Geometry: final body of the model. Coordinates: model frame, mm. Face numbers are marked on the shaded views. Coordinates: 2 decimals unless noted, no trailing zeros. Write each loop counter-clockwise with the first axis right and the second up, starting at its lowest first coordinate (ties: lowest second). Pieces come first, ordered by that corner, then holes.
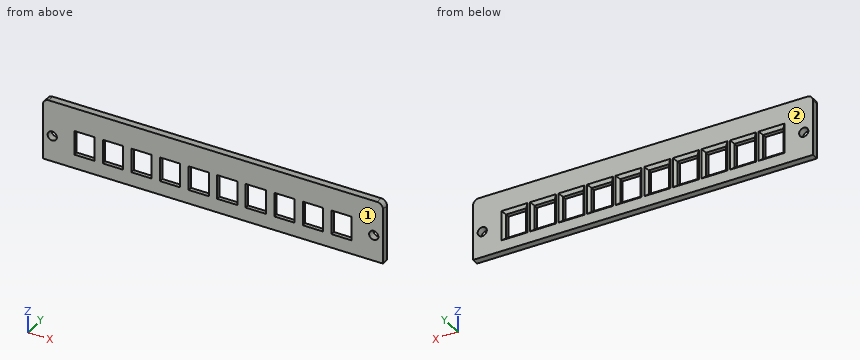
Autodesk Inventor part; units mm, degrees
ref_plane "YZ Plane" through (0, 0, 0) normal (1, 0, 0) x (0, 1, 0)
ref_plane "XZ Plane" through (0, 0, 0) normal (0, 1, 0) x (-1, 0, 0)
ref_plane "XY Plane" through (0, 0, 0) normal (0, 0, 1) x (1, 0, 0)
sketch "Sketch1" plane through (0, 0, 0) normal (0, 1, 0) x (-1, 0, 0)
  line L0 (0, 0) -> (-9.9, 0)
  line L1 (0, 0) -> (0, -10.3)
  line L2 (0, -10.3) -> (-9.9, -10.3)
  line L3 (-9.9, -10.3) -> (-9.9, 0)
  line L4 (-9.9, -10.3) -> (-9.4, -10.3)
  line L5 (-9.4, -10.3) -> (-9.4, 0)
  line L6 (0, -10.3) -> (-0.5, -10.3)
  line L7 (-0.5, -10.3) -> (-0.5, 0)
  line L8 (-0.5, 0.85) -> (-9.9, 0.85)
  line L9 (-9.9, 0.85) -> (-9.9, 0)
  line L10 (0, 0) -> (0, 0.85)
  line L11 (0, 0.85) -> (-0.5, 0.85)
  line L12 (0, -10.3) -> (0, -11.15)
  line L13 (0, -11.15) -> (-9.9, -11.15)
  line L14 (-9.9, -11.15) -> (-9.9, -10.3)
  line L15 (-9.9, -11.15) -> (-19.8, -11.15)
  line L16 (-19.8, -11.15) -> (-19.8, -10.3)
  line L17 (-19.8, -10.3) -> (-19.8, 0)
  line L18 (-19.3, -10.3) -> (-19.3, 0)
  line L19 (-9.9, -10.3) -> (-19.8, -10.3)
  line L20 (-10.4, -10.3) -> (-10.4, 0)
  line L21 (-9.9, 0) -> (-9.9, -10.3)
  line L22 (-9.9, 0) -> (-9.9, 0.85)
  line L23 (-9.9, 0.85) -> (-10.4, 0.85)
  line L24 (-10.4, 0.85) -> (-19.8, 0.85)
  line L25 (-9.9, 0) -> (-19.8, 0)
  line L26 (-19.8, 0.85) -> (-19.8, 0)
  line L27 (-19.8, -11.15) -> (-29.7, -11.15)
  line L28 (-29.7, -11.15) -> (-29.7, -10.3)
  line L29 (-29.7, -10.3) -> (-29.7, 0)
  line L30 (-29.2, -10.3) -> (-29.2, 0)
  line L31 (-19.8, -10.3) -> (-29.7, -10.3)
  line L32 (-20.3, -10.3) -> (-20.3, 0)
  line L33 (-19.8, 0) -> (-19.8, -10.3)
  line L34 (-19.8, 0) -> (-19.8, 0.85)
  line L35 (-19.8, 0.85) -> (-20.3, 0.85)
  line L36 (-20.3, 0.85) -> (-29.7, 0.85)
  line L37 (-19.8, 0) -> (-29.7, 0)
  line L38 (-29.7, 0.85) -> (-29.7, 0)
  line L39 (-29.7, -11.15) -> (-39.6, -11.15)
  line L40 (-39.6, -11.15) -> (-39.6, -10.3)
  line L41 (-39.6, -10.3) -> (-39.6, 0)
  line L42 (-39.1, -10.3) -> (-39.1, 0)
  line L43 (-29.7, -10.3) -> (-39.6, -10.3)
  line L44 (-30.2, -10.3) -> (-30.2, 0)
  line L45 (-29.7, 0) -> (-29.7, -10.3)
  line L46 (-29.7, 0) -> (-29.7, 0.85)
  line L47 (-29.7, 0.85) -> (-30.2, 0.85)
  line L48 (-30.2, 0.85) -> (-39.6, 0.85)
  line L49 (-29.7, 0) -> (-39.6, 0)
  line L50 (-39.6, 0.85) -> (-39.6, 0)
  line L51 (-39.6, -11.15) -> (-49.5, -11.15)
  line L52 (-49.5, -11.15) -> (-49.5, -10.3)
  line L53 (-49.5, -10.3) -> (-49.5, 0)
  line L54 (-49, -10.3) -> (-49, 0)
  line L55 (-39.6, -10.3) -> (-49.5, -10.3)
  line L56 (-40.1, -10.3) -> (-40.1, 0)
  line L57 (-39.6, 0) -> (-39.6, -10.3)
  line L58 (-39.6, 0) -> (-39.6, 0.85)
  line L59 (-39.6, 0.85) -> (-40.1, 0.85)
  line L60 (-40.1, 0.85) -> (-49.5, 0.85)
  line L61 (-39.6, 0) -> (-49.5, 0)
  line L62 (-49.5, 0.85) -> (-49.5, 0)
  line L63 (-49.5, -11.15) -> (-59.4, -11.15)
  line L64 (-59.4, -11.15) -> (-59.4, -10.3)
  line L65 (-59.4, -10.3) -> (-59.4, 0)
  line L66 (-58.9, -10.3) -> (-58.9, 0)
  line L67 (-49.5, -10.3) -> (-59.4, -10.3)
  line L68 (-50, -10.3) -> (-50, 0)
  line L69 (-49.5, 0) -> (-49.5, -10.3)
  line L70 (-49.5, 0) -> (-49.5, 0.85)
  line L71 (-49.5, 0.85) -> (-50, 0.85)
  line L72 (-50, 0.85) -> (-59.4, 0.85)
  line L73 (-49.5, 0) -> (-59.4, 0)
  line L74 (-59.4, 0.85) -> (-59.4, 0)
  line L75 (-59.4, -11.15) -> (-69.3, -11.15)
  line L76 (-69.3, -11.15) -> (-69.3, -10.3)
  line L77 (-69.3, -10.3) -> (-69.3, 0)
  line L78 (-68.8, -10.3) -> (-68.8, 0)
  line L79 (-59.4, -10.3) -> (-69.3, -10.3)
  line L80 (-59.9, -10.3) -> (-59.9, 0)
  line L81 (-59.4, 0) -> (-59.4, -10.3)
  line L82 (-59.4, 0) -> (-59.4, 0.85)
  line L83 (-59.4, 0.85) -> (-59.9, 0.85)
  line L84 (-59.9, 0.85) -> (-69.3, 0.85)
  line L85 (-59.4, 0) -> (-69.3, 0)
  line L86 (-69.3, 0.85) -> (-69.3, 0)
  line L87 (-69.3, -11.15) -> (-79.2, -11.15)
  line L88 (-79.2, -11.15) -> (-79.2, -10.3)
  line L89 (-79.2, -10.3) -> (-79.2, 0)
  line L90 (-78.7, -10.3) -> (-78.7, 0)
  line L91 (-69.3, -10.3) -> (-79.2, -10.3)
  line L92 (-69.8, -10.3) -> (-69.8, 0)
  line L93 (-69.3, 0) -> (-69.3, -10.3)
  line L94 (-69.3, 0) -> (-69.3, 0.85)
  line L95 (-69.3, 0.85) -> (-69.8, 0.85)
  line L96 (-69.8, 0.85) -> (-79.2, 0.85)
  line L97 (-69.3, 0) -> (-79.2, 0)
  line L98 (-79.2, 0.85) -> (-79.2, 0)
  line L99 (-79.2, -11.15) -> (-89.1, -11.15)
  line L100 (-89.1, -11.15) -> (-89.1, -10.3)
  line L101 (-89.1, -10.3) -> (-89.1, 0)
  line L102 (-88.6, -10.3) -> (-88.6, 0)
  line L103 (-79.2, -10.3) -> (-89.1, -10.3)
  line L104 (-79.7, -10.3) -> (-79.7, 0)
  line L105 (-79.2, 0) -> (-79.2, -10.3)
  line L106 (-79.2, 0) -> (-79.2, 0.85)
  line L107 (-79.2, 0.85) -> (-79.7, 0.85)
  line L108 (-79.7, 0.85) -> (-89.1, 0.85)
  line L109 (-79.2, 0) -> (-89.1, 0)
  line L110 (-89.1, 0.85) -> (-89.1, 0)
  line L111 (-89.1, -11.15) -> (-99, -11.15)
  line L112 (-99, -11.15) -> (-99, -10.3)
  line L113 (-99, -10.3) -> (-99, 0)
  line L114 (-98.5, -10.3) -> (-98.5, 0)
  line L115 (-89.1, -10.3) -> (-99, -10.3)
  line L116 (-89.6, -10.3) -> (-89.6, 0)
  line L117 (-89.1, 0) -> (-89.1, -10.3)
  line L118 (-89.1, 0) -> (-89.1, 0.85)
  line L119 (-89.1, 0.85) -> (-89.6, 0.85)
  line L120 (-89.6, 0.85) -> (-99, 0.85)
  line L121 (-89.1, 0) -> (-99, 0)
  line L122 (-99, 0.85) -> (-99, 0)
  line L123 (0, -11.15) -> (0, 0.85)
  line L124 (0, -11.15) -> (0, -14.15)
  line L125 (0, -14.15) -> (0, -14.15)
  line L126 (-99, 0.85) -> (-102, 0.85)
  line L127 (-102, 0.85) -> (-102, 3.85)
  line L128 (0, -14.15) -> (-102, -14.15)
  line L129 (-102, -14.15) -> (-102, 3.85)
  line L130 (0, 3.89) -> (0, -14.15)
  line L131 (0, -11.15) -> (0, -11.15)
  line L132 (0, 0.85) -> (0, 0.85)
  line L133 (0, -11.15) -> (-2, -11.15)
  line L134 (-2, -11.15) -> (-2, 0.85)
  line L135 (0, -14.15) -> (3.2, -14.15)
  line L136 (3.2, -14.15) -> (3.2, 3.89)
  line L137 (3.2, 3.89) -> (0, 3.89)
  line L138 (0, -11.15) -> (3.2, -11.15)
  line L139 (0, 0.85) -> (3.2, 0.85)
  line L140 (3.2, -14.15) -> (6.2, -14.15)
  line L141 (6.2, 3.89) -> (3.2, 3.89)
  line L142 (0, -14.15) -> (6.2, -14.15)
  line L143 (-49.5, 3.85) -> (-49.5, 0.85)
  line L144 (6.2, 3.89) -> (6.2, 7.09)
  line L145 (6.2, 7.09) -> (6.2, 13.49)
  line L146 (3.2, 3.89) -> (3.2, 13.45)
  line L147 (-102, 3.85) -> (-102, 13.45)
  line L148 (0, 3.89) -> (0, 13.49)
  line L149 (-49.5, 3.85) -> (-87.8335, 3.85)
  line L150 (-49.5, 3.85) -> (-11.1665, 3.89)
  line L151 (-11.1665, 3.89) -> (0, 3.89)
  line L152 (-87.8335, 3.85) -> (-102, 3.85)
  line L153 (-102, -14.15) -> (-105, -14.15)
  line L154 (-105, 13.49) -> (6.2, 13.49)
  line L155 (6.2, 7.09) -> (-105, 7.09)
  line L156 (-49.5, 3.85) -> (-49.5, 7.09)
  line L157 (-49.5, 7.09) -> (-49.5, 10.29)
  line L158 (-49.5, 10.29) -> (-11.1665, 10.29)
  line L159 (-49.5, 10.29) -> (-87.8335, 10.29)
  line L160 (-91.0335, 13.49) -> (-84.6335, 13.49)
  line L161 (-84.6335, 13.49) -> (-84.6335, 7.09)
  line L162 (-84.6335, 7.09) -> (-91.0335, 7.09)
  line L163 (-91.0335, 7.09) -> (-91.0335, 13.49)
  line L164 (-91.0335, 13.49) -> (-84.6335, 7.09) construction
  line L165 (-84.6335, 13.49) -> (-91.0335, 7.09) construction
  line L166 (-14.3665, 13.49) -> (-7.9665, 13.49)
  line L167 (-7.9665, 13.49) -> (-7.9665, 7.09)
  line L168 (-7.9665, 7.09) -> (-14.3665, 7.09)
  line L169 (-14.3665, 7.09) -> (-14.3665, 13.49)
  line L170 (-14.3665, 13.49) -> (-7.9665, 7.09) construction
  line L171 (-7.9665, 13.49) -> (-14.3665, 7.09) construction
  circle A0 centre (-11.1665, 10.29) radius 1.6
  circle A1 centre (-87.8335, 10.29) radius 1.6
  line L172 (6.2, -14.15) -> (9.4, -14.15)
  line L173 (9.4, -14.15) -> (9.4, 3.89)
  line L174 (9.4, 3.89) -> (6.2, 3.89)
  line L175 (9.4, 3.89) -> (9.4, 7.09)
  line L176 (9.4, 7.09) -> (6.2, 7.09)
  line L177 (-105, 7.09) -> (-108.2, 7.09)
  line L178 (-108.2, -14.15) -> (-105, -14.15)
  line L179 (-105, 13.49) -> (-105, 7.09)
  line L180 (-102, -14.15) -> (-108.4, -14.15)
  line L181 (-108.4, -14.15) -> (-108.4, 7.09)
  line L182 (-108.4, 7.09) -> (-108.2, 7.09)
  line L183 (-108.4, -5.13) -> (-105.2, -5.13)
  line L184 (3.2, -11.15) -> (3.2, 0.85)
  line L185 (3.2, -5.15) -> (9.4, -5.15)
  line L186 (3.2, -5.15) -> (9.4, -5.15) construction
  line L187 (9.4, -5.15) -> (6.2, -5.15)
  circle A2 centre (6.2, -5.15) radius 1.6
  circle A3 centre (-105.2, -5.15) radius 1.6
  line L188 (0, 0) -> (-9.9, 0)
  line L189 (-4.95, 0) -> (-4.95, -10.3)
  line L190 (-8.45, -0.95) -> (-1.45, -0.95)
  line L191 (-1.45, -0.95) -> (-1.45, -9.35)
  line L192 (-1.45, -9.35) -> (-8.45, -9.35)
  line L193 (-8.45, -9.35) -> (-8.45, -0.95)
  line L194 (-8.45, -0.95) -> (-1.45, -9.35) construction
  line L195 (-1.45, -0.95) -> (-8.45, -9.35) construction
  line L196 (-9.4, 0) -> (-0.5, 0)
  point P0 (-2, 0)
  point P1 (-2, -10.3)
  point P2 (0, 0.85)
  point P3 (0, 7.09)
  point P4 (3.2, 7.09)
  point P5 (-4.95, -5.15)
  dimension "d0" = 9.9
  dimension "d1" = 10.3
  dimension "d2" = 0.5
  dimension "d3" = 0.5
  dimension "d6" = 0.85
  dimension "d7" = 0.85
  dimension "d10" = 9.9
  dimension "d15" = 3
  dimension "d16" = 0
  dimension "d19" = 3
  dimension "d20" = 2
  dimension "d30" = 3.2
  dimension "d31" = 3
  dimension "d32" = 3
  dimension "d35" = 3.2
  dimension "d36" = 6.4
  dimension "d38" = 38.3335
  dimension "d45" = 3.2
  dimension "d47" = 38.3335
  dimension "d48" = 6.4
  dimension "d49" = 6.4
  dimension "d50" = 3.2
  dimension "d51" = 3.2
  dimension "d53" = 6.4
  dimension "d58" = 3.2
  dimension "d59" = 3.2
  dimension "d60" = 3.2
  dimension "d63" = 7
  dimension "d64" = 8.4
  dimension "d72" = 8.9
extrude "Extrusion6" add sketch "Sketch1" along normal blind 2.4 contours L1 L2 L7 L0 | L10 L139 L136 L138 L12 L1 | L0 L134 L8 L11 L10 | L7 L2 L134 L192 L191 L190 L0 | L12 L13 L134 L2 | L11 L8 L23 L24 L35 L36 L47 L48 L59 L60 L143 L150 L151 L130 | L130 L137 L136 L139 | L134 L190 L189 L0 | L0 L9 L8 L134 | L124 L128 L129 L126 L122 L113 L112 L111 L99 L87 L75 L63 L51 L39 L27 L15 L13 | L138 L136 L135 L124 | L148 L155 L146 L137 | L151 L150 L156 L155 L148 | L136 L141 L174 L173 L185 A2 | L189 L190 L193 L192 L2 L5 L0 | L190 L191 L192 L134 | L134 L192 L189 L190 | L134 L13 L14 L2 | L2 L189 L192 L134 | L136 L185 A2 L173 L172 L140 | L146 L155 L144 L141 | L5 L2 L3 L0 | L189 L192 L193 L190 | L9 L25 L26 L24 L23 | L15 L16 L19 L14 | L153 L178 L180 L181 L182 L177 L155 L147 L127 L129 | L144 L176 L175 L174 | L143 L71 L72 L83 L84 L95 L96 L107 L108 L119 L120 L126 L127 L152 L149 | L149 L152 L147 L155 L156 | L3 L19 L20 L25 | L27 L28 L31 L16 | L60 L59 L50 L61 L62 | L62 L73 L74 L72 L71 | L20 L19 L18 L25 | L26 L37 L38 L36 L35 | L31 L32 L37 L17 | L17 L25 L18 L19 | L39 L40 L43 L28 | L120 L119 L110 L121 L122 | L61 L54 L55 L53 | L53 L67 L68 L73 | L31 L30 L37 L32 | L43 L44 L49 L29 | L29 L37 L30 L31 | L51 L52 L55 L40 | L121 L114 L115 L113 | L48 L47 L38 L49 L50 | L52 L63 L64 L67 | L61 L56 L55 L54 | L68 L67 L66 L73 | L74 L85 L86 L84 L83 | L43 L42 L49 L44 | L55 L56 L61 L41 | L41 L49 L42 L43 | L108 L107 L98 L109 L110 | L115 L100 L111 L112 | L121 L116 L115 L114 | L66 L67 L65 L73 | L65 L79 L80 L85 | L75 L76 L79 L64 | L109 L102 L103 L101 | L101 L115 L116 L121 | L80 L79 L78 L85 | L86 L97 L98 L96 L95 | L87 L88 L91 L76 | L103 L88 L99 L100 | L109 L104 L103 L102 | L78 L79 L77 L85 | L77 L91 L92 L97 | L97 L90 L91 L89 | L89 L103 L104 L109 | L92 L91 L90 L97
extrude "Extrusion7" cut sketch "Sketch1" along normal through all contours L190 L191 L192 L134 | L134 L192 L189 L190 | L189 L192 L193 L190
chamfer "Chamfer2" distance 1 angle 45 4 edges at (4.95, 2.4, -9.35) (1.45, 2.4, -5.15) (8.45, 2.4, -5.15) (4.95, 2.4, -0.95)
pattern_linear "Rectangular Pattern2" count 10 spacing 9.9 along (1, 0, 0) of "Extrusion7", "Chamfer2"
fillet "Fillet1" radius 2 2 edges at (108.4, 1.2, 7.09) (-9.4, 1.2, 7.09)
properties part number "10x led strip holder top cover"
Item 1: Pin query (flat end, axial travel): pin 1 (2.5 mm diameter, centred on x = -6.2, z = -5.15, fed in from +Y); pin 2 (2 mm diameter, centred on x = 21.5, z = -7.5, fed in from +Y). Return the tip coordinate at first contact, or that it passes through.
Derived:
pin 1: passes through
pin 2: stops at y = 2.15
Item 2: Section A-A, the plane x = 105.2. Output: boundary loops of the cut face in (y, z), plus the area to 3 significant figures.
Derived:
outline: (0, -14.15) - (2.4, -14.15) - (2.4, -6.75) - (0, -6.75) - close; (0, -3.55) - (2.4, -3.55) - (2.4, 7.09) - (0, 7.09) - close
area: 43.3 mm2
Item 3: Material intervals for probe 1 along Z at (x, y) = (-6.2, 0.85); probe 2 along Z at (x, y) = (6, 1.05); probe 3 along Y at (x, z) = (5, 0), sorted ascending.
Derived:
probe 1: z = -14.15 to -6.75, -3.55 to 7.09
probe 2: z = -14.15 to -9.35, -0.95 to 7.09
probe 3: y = 0 to 2.35
Item 4: Section B-B, the plane z = -2.5. State how many separate pieces and enclosed holes the cut face has, plus the area to 3 significant figures.
Derived:
separate pieces: 11
enclosed holes: 0
area: 105 mm2
Item 5: Pull-direction query (Y, two-part tool) for the marked faces 1 and 2; classes: released by +Y, released by -Y, zero draft, split by the parting line, or undercut.
Derived:
face 1: released by -Y
face 2: released by +Y
Item 6: Section D-D, the plane x = 7. Output: boundary loops of the cut face in (y, z).
Derived:
outline: (0, -14.15) - (2.4, -14.15) - (2.4, -10.35) - (1.4, -9.35) - (0, -9.35) - close; (0, -0.95) - (1.4, -0.95) - (2.4, 0.05) - (2.4, 7.09) - (0, 7.09) - close
